Here's how the part is built. I have some questions about the finished solid (model axes, mm). A direction names the side the tool comes from. Give positions to 0.01 mm unless a question says otherwise; leave off trailing zeros. Loops run counter-clockwise (first coordinate to the right, second up) from the corner with the lowest first, then second, coordinate; pieces in that order, holes last. Notation, with made-up numbers: (67.5, 68) - (80.5, 68) arc R19 cw to (80.5, 75) - close; hole circle Ø8 at (61, -26.75). An arc over 180 degrees is marked (long way). Return JSON: item names as keys, results as strings. Group by question number.
(1) If we mould it in two halves opening along Z, with no side actions, what happens to faces 1 (the cylindrical face through (2, 23, 17)), 2 (the flat face through (1, -6, -5.058)), 3 (the flat face through (3, 5, 3)), 4 (the flat face through (1, 12, 0))? For each: released by +Z, released by -Z, zero draft, split by the parting line, or undercut.
(2) If we section it at A-A (y = 6): Please give me the cut outline in (x, z), then the cut area to 3 significant figures.
(3) If we section it at D-D (z = 4): Please give me the cut outline in (x, y).
(4) If we section it at C-C (x = 1.05): Please give me the cut outline in (y, z).
(5) On a 3-axis mill with a long thin cutter (end or side, diameter ignored), from which of +Z, -Z, +X, -X, +Y, -Y can I reach the whole of each face in a straight line? I mean faces 5 (the flat face through (1, 2.251, -2)), 6 (the flat face through (1, 4.251, -3)), 7 (the flat face through (1, 20.398, -9)), 8 (the flat face through (1, -15.498, 9)). Say none if no direction works.
(6) If we section it at B-B (y = 10.5): Please give me the cut outline in (x, z), then the cut area to 3 significant figures.
(7) I need wall thicknesses on probe 1 along Z at (x, y) = (1.15, 10.5); probe 2 along Z at (x, y) = (1.35, -8); probe 3 along Y at (x, z) = (1.5, 14). Which ranges of each line are inside material? Lowest first, please. Write a range as [from, to].
(8) For P1, Ø5.5, axis at y = 19.5, z = 14, coming from the -X side; P2, Ø1.5, axis at x = 1.5, z = -7.5, coming from the -Y side; P3, Ø0.9, axis at x = 2, z = -10.5, coming from the +Y side, each with a flat end and sliding along its axis, tell me the tip position at first contact or that it passes through.
```python
from build123d import *

# Parameters (mm, degrees)
T_LE_DE_BASE_PLI_E1_DEPTH    = 18
ENL_V_MAT_EXTRU_1_DEPTH      = 36.185224172
ENL_V_MAT_EXTRU_1_DEPTH_BACK = 36.185224172
ESQUISSE6_R                  = 1.65
ENL_V_MAT_EXTRU_2_DEPTH      = 35.756294394
ENL_V_MAT_EXTRU_2_DEPTH_BACK = 35.756294394
ESQUISSE7_R                  = 1.65
CONG_1_R                     = 5
BOSS_EXTRU_1_OUTLINE_R       = 1.65
BOSS_EXTRU_1_DEPTH           = 17
BOSS_EXTRU_1_START           = -3
BOSS_EXTRU_1_2_OUTLINE_R     = 1.65
BOSS_EXTRU_1_2_DEPTH         = 3


with BuildPart() as part:
    # Tôle de base pliée1: sheet metal written as solids
    # Esquisse1 → Tôle de base pliée1 (new body)
    with BuildSketch(Plane.XY):
        with BuildLine():
            Line((20, 0), (5, 0))
            ThreePointArc((5, 0), (1.464466094, 1.464466094), (0, 5))
            Line((0, 5), (0, 25))
            Line((0, 25), (3, 25))
            Line((3, 25), (3, 5))
            ThreePointArc((3, 5), (3.585786438, 3.585786438), (5, 3))
            Line((5, 3), (20, 3))
            Line((20, 3), (20, 0))
        make_face()
    extrude(amount=T_LE_DE_BASE_PLI_E1_DEPTH)

    # Esquisse6 → Enlèv. mat.-Extru.1 (cut, two sides: drawn at the far end of the back side and taken through both)
    with BuildSketch(Plane(origin=(3, 0, 0), x_dir=(0, 0, -1), z_dir=(1, 0, 0)).offset(-ENL_V_MAT_EXTRU_1_DEPTH_BACK)):
        with Locations((-14, 19.5)):
            Circle(ESQUISSE6_R)
        with Locations(Location((-14, 10.5, 0), (0, 0, 180))):
            Circle(ESQUISSE6_R)
    extrude(amount=ENL_V_MAT_EXTRU_1_DEPTH + ENL_V_MAT_EXTRU_1_DEPTH_BACK, mode=Mode.SUBTRACT)

    # Esquisse7 → Enlèv. mat.-Extru.2 (cut, two sides: drawn at the far end of the back side and taken through both)
    with BuildSketch(Plane(origin=(0, 3, 0), x_dir=(1, 0, 0), z_dir=(0, 1, 0)).offset(-ENL_V_MAT_EXTRU_2_DEPTH_BACK)):
        with Locations(Location((12.5, -4, 0), (0, 0, 270))):
            Circle(ESQUISSE7_R)
        with Locations(Location((12.5, -14, 0), (0, 0, 90))):
            Circle(ESQUISSE7_R)
    extrude(amount=ENL_V_MAT_EXTRU_2_DEPTH + ENL_V_MAT_EXTRU_2_DEPTH_BACK, mode=Mode.SUBTRACT)

    # Congé1
    cong_1_edges = [part.edges().sort_by_distance(p)[0] for p in [
        (20, 1.5, 18),
        (1.5, 25, 18),
        (20, 1.5, 0),
        (1.5, 25, 0),
    ]]
    fillet(cong_1_edges, radius=CONG_1_R)

    # Boss.-Extru.1: read off the stored shape, not the designer's step
    # Boss.-Extru.1 outline → Boss.-Extru.1 (cut)
    with BuildSketch(Plane(origin=(3, 0, 0), x_dir=(0, 0, -1), z_dir=(1, 0, 0))):
        with BuildLine():
            Line((-13, -15.497787144), (-5, -15.497787144))
            ThreePointArc((-5, -15.497787144), (-1.464466094, -14.03332105), (0, -10.497787144))
            Line((0, -10.497787144), (0, 2.251106428))
            Line((0, 2.251106428), (5.057824139, 2.251106428))
            Line((5.057824139, 2.251106428), (5.057824139, -13.661822952))
            Line((5.057824139, -13.661822952), (13.362072183, -13.661822952))
            Line((13.362072183, -13.661822952), (13.362072183, 20.398028744))
            Line((13.362072183, 20.398028744), (5.057824139, 20.398028744))
            Line((5.057824139, 20.398028744), (5.057824139, 4.251106428))
            Line((5.057824139, 4.251106428), (0, 4.251106428))
            Line((0, 4.251106428), (0, 20))
            ThreePointArc((0, 20), (-1.464466094, 23.535533906), (-5, 25))
            Line((-5, 25), (-13, 25))
            ThreePointArc((-13, 25), (-16.535533906, 23.535533906), (-18, 20))
            Line((-18, 20), (-18, -10.497787144))
            ThreePointArc((-18, -10.497787144), (-16.535533906, -14.03332105), (-13, -15.497787144))
        make_face()
        with Locations((-14, -7.997787144)):
            Circle(BOSS_EXTRU_1_OUTLINE_R, mode=Mode.SUBTRACT)
        with Locations((-4, -7.997787144)):
            Circle(BOSS_EXTRU_1_OUTLINE_R, mode=Mode.SUBTRACT)
        with Locations((-14, 10.5)):
            Circle(BOSS_EXTRU_1_OUTLINE_R, mode=Mode.SUBTRACT)
        with Locations((-14, 19.5)):
            Circle(BOSS_EXTRU_1_OUTLINE_R, mode=Mode.SUBTRACT)
    extrude(amount=BOSS_EXTRU_1_DEPTH, mode=Mode.SUBTRACT)

    # Boss.-Extru.1 2 outline → Boss.-Extru.1 2 (add)
    with BuildSketch(Plane(origin=(3, 0, 0), x_dir=(0, 0, -1), z_dir=(1, 0, 0)).offset(BOSS_EXTRU_1_START)):
        with BuildLine():
            Line((-13, -15.497787144), (-5, -15.497787144))
            ThreePointArc((-5, -15.497787144), (-1.464466094, -14.03332105), (0, -10.497787144))
            Line((0, -10.497787144), (0, 2.251106428))
            Line((0, 2.251106428), (5.057824139, 2.251106428))
            Line((5.057824139, 2.251106428), (5.057824139, -13.661822952))
            Line((5.057824139, -13.661822952), (13.362072183, -13.661822952))
            Line((13.362072183, -13.661822952), (13.362072183, 20.398028744))
            Line((13.362072183, 20.398028744), (5.057824139, 20.398028744))
            Line((5.057824139, 20.398028744), (5.057824139, 4.251106428))
            Line((5.057824139, 4.251106428), (0, 4.251106428))
            Line((0, 4.251106428), (0, 20))
            ThreePointArc((0, 20), (-1.464466094, 23.535533906), (-5, 25))
            Line((-5, 25), (-13, 25))
            ThreePointArc((-13, 25), (-16.535533906, 23.535533906), (-18, 20))
            Line((-18, 20), (-18, -10.497787144))
            ThreePointArc((-18, -10.497787144), (-16.535533906, -14.03332105), (-13, -15.497787144))
        make_face()
        with Locations((-14, -7.997787144)):
            Circle(BOSS_EXTRU_1_2_OUTLINE_R, mode=Mode.SUBTRACT)
        with Locations((-4, -7.997787144)):
            Circle(BOSS_EXTRU_1_2_OUTLINE_R, mode=Mode.SUBTRACT)
        with Locations((-14, 10.5)):
            Circle(BOSS_EXTRU_1_2_OUTLINE_R, mode=Mode.SUBTRACT)
        with Locations((-14, 19.5)):
            Circle(BOSS_EXTRU_1_2_OUTLINE_R, mode=Mode.SUBTRACT)
    extrude(amount=BOSS_EXTRU_1_2_DEPTH)


solid = part.part
```
Values:
{
 "1": {"face 1": "released by +Z", "face 2": "undercut", "face 3": "zero draft", "face 4": "undercut"},
 "2": {"outline": "(0, -13.36) - (3, -13.36) - (3, -5.06) - (0, -5.06) - close; (0, 0) - (3, 0) - (3, 18) - (0, 18) - close", "area": "78.9 mm2"},
 "3": {"outline": "(0, -15.4) - (3, -15.4) - (3, -9.65) - (0, -9.65) - close; (0, -6.35) - (3, -6.35) - (3, 24.9) - (0, 24.9) - close"},
 "4": {"outline": "(-15.5, 5) arc R5 ccw to (-10.5, 0) - (2.25, 0) - (2.25, -5.06) - (-13.66, -5.06) - (-13.66, -13.36) - (20.4, -13.36) - (20.4, -5.06) - (4.25, -5.06) - (4.25, 0) - (20, 0) arc R5 ccw to (25, 5) - (25, 13) arc R5 ccw to (20, 18) - (-10.5, 18) arc R5 ccw to (-15.5, 13) - close; hole circle Ø3.3 at (-8, 4); hole circle Ø3.3 at (-8, 14); hole circle Ø3.3 at (10.5, 14); hole circle Ø3.3 at (19.5, 14)"},
 "5": {"face 5": "+X, -X, -Y", "face 6": "+X, -X, +Y", "face 7": "-Z, +X, -X, +Y", "face 8": "+Z, -Z, +X, -X, -Y"},
 "6": {"outline": "(0, -13.36) - (3, -13.36) - (3, -5.06) - (0, -5.06) - close; (0, 0) - (3, 0) - (3, 12.35) - (0, 12.35) - close; (0, 15.65) - (3, 15.65) - (3, 18) - (0, 18) - close", "area": "69.0 mm2"},
 "7": {"probe 1": "[-13.36, -5.06], [0, 12.35], [15.65, 18]", "probe 2": "[-13.36, -5.06], [0, 2.35], [5.65, 12.35], [15.65, 18]", "probe 3": "[-15.4, -9.65], [-6.35, 8.85], [12.15, 17.85], [21.15, 24.9]"},
 "8": {"P1": "x = 0", "P2": "y = -13.66", "P3": "y = 20.4"}
}
